Geometry check sheet. Reference: the model listing, model coordinates, mm. A direction names the side the tool comes from. Give positions to 0.01 mm unless a question says otherwise; leave off trailing zeros. Write each loop counter-clockwise with the first axis right and the second up, starting at its lowest first coordinate (ties: lowest second). Pieces come first, ordered by that corner, then holes. Notation, with made-up numbers: (31.5, 17.5) - (78.5, 17.5) arc R27 cw to (78.5, 38.5) - close; hole circle Ø7 at (11, 87). An arc over 180 degrees is marked (long way). Use a Markdown table: item, result.
```python
from build123d import *

# Parameters (mm, degrees)
F1_DEPTH = 381
F0_R     = 127
F2_DEPTH = 38.1
F0_R_2   = 152.4
F3_DEPTH = 19.05
F4_R     = 25.4


with BuildPart() as f1:
    # F0 (on Top) → F1 (new body)
    with BuildSketch(Plane.XY):
        Polygon((64.913587, 4.291234), (45.863587, 23.341234), (-17.636413, 23.341234), (-44.577181, 23.349866), (-89.478462, -21.551415), (-108.534565, -40.595311), (-108.534565, -104.095311), (-108.543197, -131.03608), (-63.641916, -175.93736), (-44.59802, -194.993464), (18.90198, -194.993464), (45.85138, -194.993464), (90.752661, -150.092183), (109.802658, -131.029975), (109.802658, -67.529975), (109.814868, -40.610047), align=None)
        Polygon((-89.478462, -48.500815), (-36.686413, 4.291234), (-17.636413, 4.291234), (37.937591, 4.289049), (90.752661, -48.492183), (90.748342, -85.846952), (90.744029, -123.151415), (37.958084, -175.93736), (-36.692516, -175.93736), (-89.478462, -123.151415), (-89.478462, -85.826115), align=None, mode=Mode.SUBTRACT)
    extrude(amount=F1_DEPTH)

    # F0 (on Top) → F2 (join)
    with BuildSketch(Plane.XY):
        with Locations((0, -85.83646)):
            Circle(F0_R)
        Polygon((-17.636413, 23.341234), (45.863587, 23.341234), (64.913587, 4.291234), (109.814868, -40.610047), (109.802658, -67.529975), (109.802658, -131.029975), (90.752661, -150.092183), (45.85138, -194.993464), (18.90198, -194.993464), (-44.59802, -194.993464), (-63.641916, -175.93736), (-108.543197, -131.03608), (-108.534565, -104.095311), (-108.534565, -40.595311), (-89.478462, -21.551415), (-44.577181, 23.349866), align=None, mode=Mode.SUBTRACT)
    extrude(amount=F2_DEPTH)

    # F0 (on Top) → F3 (join)
    with BuildSketch(Plane.XY):
        with Locations((0, -85.83646)):
            Circle(F0_R_2)
        with Locations((0, -85.83646)):
            Circle(F0_R, mode=Mode.SUBTRACT)
    extrude(amount=F3_DEPTH)

    # F4
    f4_edges = [f1.edges().sort_by_distance(p)[0] for p in [
        (-89.478462, -85.826115, 0),
        (-63.085489, -149.544388, 0),
        (-63.082437, -22.10479, 0),
        (-27.161413, 4.291234, 0),
        (10.150589, 4.290141, 0),
        (0.632784, -175.93736, 0),
        (64.351056, -149.544388, 0),
        (90.748345, -85.821799, 0),
        (64.345126, -22.101567, 0),
    ]]
    fillet(f4_edges, radius=F4_R)


solid = f1.part
```
1) Set-up check for faces 1 (the flat face through (-57, 28, 19.05)), 2 (the cylindrical face through (-68.01, -16.23, 7.24)), 3 (the flat face through (63.975, -21.732, 200.711)): record each of +Z, -Z, +X, -X, +Y, -Y from which the full face is reachable in a straight line by a thin tool's end or side.
Working result:
| item | result |
|---|---|
| face 1 | +Z |
| face 2 | -Z |
| face 3 | +Z, -Z |
2) Mould release check, pull along Y, two halves, no side actions. Record for faces 4 (the flat face through (64.721, -149.175, 200.711)), 5 (the flat face through (65, -150, 381)), 6 (the cylindrical face through (-0.04, -183.58, 7.24)), 7 (the cylindrical face through (121.135, -47.689, 28.442)): pulls with the +Y half, pulls with the -Y half, needs draft (parallel to the pull), parting line crosses it, or undercut.
Working result:
| item | result |
|---|---|
| face 4 | undercut |
| face 5 | needs draft |
| face 6 | undercut |
| face 7 | parting line crosses it |
3) Depth check by flat-ended pin: P1, Ø8, axis at x = -77.5, z = 283.5, coming from the +Y side; P2, Ø10, axis at y = -189, z = 116.5, coming from the +X side; P3, Ø6, axis at y = -3.5, z = 115.5, coming from the -X side. Enter the tip coordinate at first touch or a pass-through.
Working result:
| item | result |
|---|---|
| P1 | stops at y = -5.57 |
| P2 | stops at x = 56.84 |
| P3 | stops at x = -74.43 |
4) Material ranges on L1, parallel to Y at x = -18.5, z = 294.5; L2, parallel to X at y = -108, z = 329; L3, parallel to X at y = -65, z = 98, recorded low to high. Write a range as from..to.
Working result:
| item | result |
|---|---|
| L1 | y = -194.99..-175.94, 4.29..23.34 |
| L2 | x = -108.54..-89.48, 90.75..109.8 |
| L3 | x = -108.53..-89.48, 90.75..109.8 |
5) Section check B-B on y = -217.5. Record the boundary of the cut face in (x, z).
Working result:
| item | result |
|---|---|
| outline | (-76.75, 0) - (76.75, 0) - (76.75, 19.05) - (-76.75, 19.05) - close |
6) Section check A-A on z = 341. Record the boundary of the cut face in (x, y), then the cut area to 3 significant figures.
Working result:
| item | result |
|---|---|
| outline | (-108.54, -131.04) - (-63.64, -175.94) - (-44.6, -194.99) - (45.85, -194.99) - (90.75, -150.09) - (109.8, -131.03) - (109.8, -67.53) - (109.81, -40.61) - (45.86, 23.34) - (-17.64, 23.34) - (-44.58, 23.35) - (-89.48, -21.55) - (-108.53, -40.6) - (-108.53, -104.1) - close; hole (-89.48, -123.15) - (-36.69, -175.94) - (37.96, -175.94) - (90.74, -123.15) - (90.75, -48.49) - (37.94, 4.29) - (-17.64, 4.29) - (-36.69, 4.29) - (-89.48, -48.5) - close |
| area | 12,600 mm² |
